Geometry: final body of the model. Coordinates: model frame, mm. Coordinates: 2 decimals unless noted, no trailing zeros. Write each loop counter-clockwise with the first axis right and the second up, starting at its lowest first coordinate (ties: lowest second). Pieces come first, ordered by that corner, then holes. Notation, with made-up numbers: (49.25, -31.5) -> (95.25, -31.5) arc R25 cw to (95.25, -10.5) -> close; hole circle Ø2 at (65.5, 86). An arc over 180 degrees is marked (long way). One line per item, written item: value.
```python
from build123d import *

# Parameters (mm, degrees)
SKETCH1_W           = 250
SKETCH1_H           = 127
BOSS_EXTRUDE1_DEPTH = 6.35
SKETCH2_R           = 6.35
SKETCH2_R_2         = 3.175
SKETCH2_R_3         = 9.525
CUT_EXTRUDE1_DEPTH  = 281.480520714


with BuildPart() as part:
    # Sketch1 → Boss-Extrude1 (new body)
    with BuildSketch(Plane(origin=(0, 0, 0), x_dir=(1, 0, 0), z_dir=(0, 1, 0))):
        with Locations((125, 63.5)):
            Rectangle(SKETCH1_W, SKETCH1_H)
    extrude(amount=BOSS_EXTRUDE1_DEPTH)

    # Sketch2 → Cut-Extrude1 (cut, through all)
    with BuildSketch(Plane(origin=(0, 6.35, 0), x_dir=(1, 0, 0), z_dir=(0, 1, 0))):
        with Locations(Location((237.3, 12.7, 0), (0, 0, 270))):
            Circle(SKETCH2_R)
        with Locations(Location((237.3, 114.3, 0), (0, 0, 270))):
            Circle(SKETCH2_R)
        with Locations(Location((12.7, 12.7, 0), (0, 0, 270))):
            Circle(SKETCH2_R)
        with Locations(Location((12.7, 114.3, 0), (0, 0, 270))):
            Circle(SKETCH2_R)
        with Locations(Location((43.193581925, 36.693581925, 0), (0, 0, 270))):
            Circle(SKETCH2_R_2)
        with Locations(Location((96.806418075, 36.693581925, 0), (0, 0, 270))):
            Circle(SKETCH2_R_2)
        with Locations(Location((96.806418075, 90.306418075, 0), (0, 0, 270))):
            Circle(SKETCH2_R_2)
        with Locations(Location((43.193581925, 90.306418075, 0), (0, 0, 270))):
            Circle(SKETCH2_R_2)
        with Locations(Location((70, 63.5, 0), (0, 0, 270))):
            Circle(SKETCH2_R_3)
    extrude(amount=-CUT_EXTRUDE1_DEPTH, mode=Mode.SUBTRACT)


solid = part.part
```
(1) Section B-B (x = 70). Return the cut outline in (y, z) (3 decimals), then the cut area to 3 significant figures.
Responses:
outline: (0, -127) -> (6.35, -127) -> (6.35, -73.025) -> (0, -73.025) -> close; (0, -53.975) -> (6.35, -53.975) -> (6.35, 0) -> (0, 0) -> close
area: 685 mm2
(2) Section C-C (x = 12.7). Return the cut outline in (y, z).
Responses:
outline: (0, -127) -> (6.35, -127) -> (6.35, -120.65) -> (0, -120.65) -> close; (0, -107.95) -> (6.35, -107.95) -> (6.35, -19.05) -> (0, -19.05) -> close; (0, -6.35) -> (6.35, -6.35) -> (6.35, 0) -> (0, 0) -> close
(3) Line query: line 1 (X direction, y = 2, z = -13.5); line 2 (Z direction, x = 237.5, y = 5.75); line 3 (X direction, y = 4.5, z = -89). Output: solid intervals per line, ascending. Write a range as [from, to].
Responses:
line 1: x = [0, 6.4], [19, 231], [243.6, 250]
line 2: z = [-127, -120.65], [-107.95, -19.05], [-6.35, 0]
line 3: x = [0, 40.3], [46.09, 93.91], [99.7, 250]
(4) Section D-D (y = 4.75). State how many separate pieces and enclosed holes the cut face has, then the cut area to 3 significant figures.
Responses:
separate pieces: 1
enclosed holes: 9
area: 30,800 mm2
(5) Section A-A (z = -63.5). Return the cut outline in (x, y) (3 decimals), then the cut area to 3 significant figures.
Responses:
outline: (0, 0) -> (60.475, 0) -> (60.475, 6.35) -> (0, 6.35) -> close; (79.525, 0) -> (250, 0) -> (250, 6.35) -> (79.525, 6.35) -> close
area: 1,470 mm2
(6) Pull-direction query (Z, two-part tool) for faces 1 (the flat face through (0, 3, -63)), 2 (the cylindrical face through (45.339, 3.219, -92.647)), 3 (the cylindrical face through (94.874, 3.219, -92.826)), 4 (the flat face through (123, 3, -127)); classes: released by +Z, released by -Z, zero draft, split by the parting line, or undercut.
Responses:
face 1: zero draft
face 2: undercut
face 3: undercut
face 4: released by -Z
